```python
from build123d import *

# Parameters (mm, degrees)
SKETCH1_W           = 508
SKETCH1_H           = 101.6
BOSS_EXTRUDE1_DEPTH = 6.35
SKETCH2_R           = 25.4
SKETCH2_R_2         = 1.651
MOTOR_MOUNT_DEPTH   = 6.35
SKETCH3_R           = 9.525
CUT_EXTRUDE2_DEPTH  = 511.573170564
SKETCH4_R           = 3.175
CUT_EXTRUDE3_DEPTH  = 511.573170564
CUT_EXTRUDE4_DEPTH  = 511.573170564


with BuildPart() as part:
    # Sketch1 → Boss-Extrude1 (new body)
    with BuildSketch(Plane.XY):
        with Locations((254, 0)):
            Rectangle(SKETCH1_W, SKETCH1_H)
    extrude(amount=-BOSS_EXTRUDE1_DEPTH)

    # Sketch2 → Motor mount (cut)
    with BuildSketch(Plane.XY):
        with Locations((40.64, 0)):
            Circle(SKETCH2_R)
        with Locations((72.39, 0)):
            Circle(SKETCH2_R_2)
        with Locations((40.64, -31.75)):
            Circle(SKETCH2_R_2)
        with Locations((8.89, 0)):
            Circle(SKETCH2_R_2)
        with Locations((40.64, 31.75)):
            Circle(SKETCH2_R_2)
    extrude(amount=-MOTOR_MOUNT_DEPTH, mode=Mode.SUBTRACT)

    # Sketch3 → Cut-Extrude2 (cut, through all)
    with BuildSketch(Plane.XY):
        with Locations((112.0775, 0)):
            Circle(SKETCH3_R)
        with Locations((183.515, 0)):
            Circle(SKETCH3_R)
        with Locations((348.615, 0)):
            Circle(SKETCH3_R)
    extrude(amount=-CUT_EXTRUDE2_DEPTH, mode=Mode.SUBTRACT)

    # Sketch4 → Cut-Extrude3 (cut, through all)
    with BuildSketch(Plane.XY):
        with Locations((9.525, 41.275)):
            Circle(SKETCH4_R)
        with Locations((9.525, -41.275)):
            Circle(SKETCH4_R)
        with Locations((498.475, 41.275)):
            Circle(SKETCH4_R)
        with Locations((498.475, -41.275)):
            Circle(SKETCH4_R)
    extrude(amount=-CUT_EXTRUDE3_DEPTH, mode=Mode.SUBTRACT)

    # Sketch7 → Cut-Extrude4 (cut, through all)
    with BuildSketch(Plane.XY):
        with BuildLine():
            Line((85.406292789, 5.08), (92.341412089, 5.08))
            ThreePointArc((92.341412089, 5.08), (96.950572969, 6.134064693), (100.643442411, 9.08671294))
            ThreePointArc((100.643442411, 9.08671294), (112.0775, 14.605), (123.511557589, 9.08671294))
            ThreePointArc((123.511557589, 9.08671294), (127.204427031, 6.134064693), (131.813587911, 5.08))
            Line((131.813587911, 5.08), (162.585112959, 5.08))
            ThreePointArc((162.585112959, 5.08), (167.45975122, 6.214203951), (171.333000793, 9.383818205))
            ThreePointArc((171.333000793, 9.383818205), (184.777760897, 15.325227036), (197.068677539, 7.263261936))
            ThreePointArc((197.068677539, 7.263261936), (202.783248212, 4.735656121), (206.626270766, 9.662753319))
            Line((206.626270766, 9.662753319), (206.626270766, 31.603209647))
            ThreePointArc((206.626270766, 31.603209647), (203.520318205, 39.101642443), (196.02188541, 42.207595003))
            Line((196.02188541, 42.207595003), (25.263102588, 42.207595003))
            ThreePointArc((25.263102588, 42.207595003), (20.881723867, 41.260150637), (17.283250038, 38.587115578))
            add(Edge.make_bspline(
                [(17.283250038, 38.587115578), (11.530533455, 32.014027317), (16.787146308, 28.551640426), (21.263438452, 31.320883809)],
                knots=[0, 0, 0, 0, 1, 1, 1, 1], degree=3))
            ThreePointArc((21.263438452, 31.320883809), (52.918543043, 34.722993545), (75.39838363, 12.177999321))
            ThreePointArc((75.39838363, 12.177999321), (79.271558889, 7.034643814), (85.406292789, 5.08))
        make_face()
    cut_extrude4 = extrude(amount=-CUT_EXTRUDE4_DEPTH, mode=Mode.SUBTRACT)

    # Mirror1: Cut-Extrude4 across plane
    add(cut_extrude4.mirror(Plane.ZX), mode=Mode.SUBTRACT)


solid = part.part
```
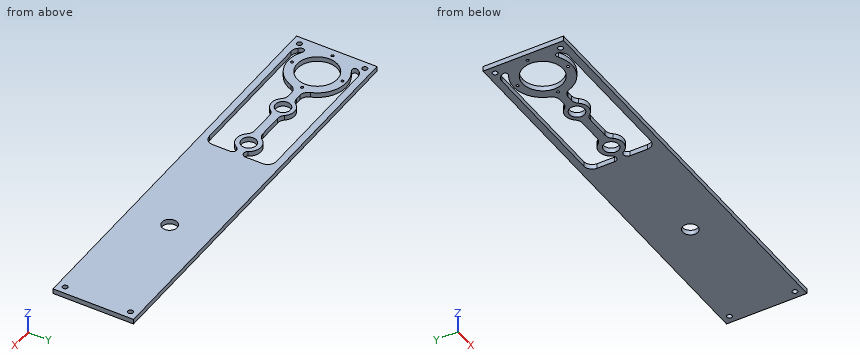
Build history of the part. All positions in model axes, mm. Coordinates: 2 decimals unless noted, no trailing zeros. Order: outer loops, then holes, each group sorted by start corner. A loop starts at its lowest first (then second) coordinate and runs counter-clockwise, first axis right, second up.
Item 1: Saw through at B-B on z = -4.5. State how many separate pieces and enclosed holes the cut face has, then the cut area to 3 significant figures.
Filled in:
separate pieces: 1
enclosed holes: 14
area: 38,500 mm2
Item 2: Drill centre lines: L1, parallel to Y at x = 40.64, z = -3.25; L2, parallel to Y at x = 79, z = -1.75; L3, parallel to Y at x = 157.5, z = -3.25. Where is each one in solid material? Low to high.
Filled in:
L1: y = -50.8 to -42.21, -36.83 to -33.4, -30.1 to -25.4, 25.4 to 30.1, 33.4 to 36.83, 42.21 to 50.8
L2: y = -50.8 to -42.21, -7.23 to 7.23, 42.21 to 50.8
L3: y = -50.8 to -42.21, -5.08 to 5.08, 42.21 to 50.8
Item 3: Saw through at A-A on x = 58. List the corners of the cut face in (y, z), then the cut area to 3 significant figures.
Filled in:
outline: (-50.8, -6.35) - (-42.21, -6.35) - (-42.21, 0) - (-50.8, 0) - close; (-32.48, -6.35) - (-18.54, -6.35) - (-18.54, 0) - (-32.48, 0) - close; (18.54, -6.35) - (32.48, -6.35) - (32.48, 0) - (18.54, 0) - close; (42.21, -6.35) - (50.8, -6.35) - (50.8, 0) - (42.21, 0) - close
area: 286 mm2
